```python
from build123d import *

# Parameters (mm, degrees)
SKETCH1_W                = 62
SKETCH1_H                = 26
BOSS_EXTRUDE1_DEPTH      = 6
SKETCH2_W                = 80
SKETCH2_H                = 10
BOSS_EXTRUDE2_DEPTH      = 50
M5_CLEARANCE_HOLE1_D     = 5.5
M5_CLEARANCE_HOLE1_DEPTH = 10
M5_CLEARANCE_HOLE1_TIP   = 1.652366702
BOSS_EXTRUDE3_DEPTH      = 9
BOSS_EXTRUDE4_START      = -80
BOSS_EXTRUDE4_DEPTH      = 9
M5_CLEARANCE_HOLE2_D     = 5.5
M5_CLEARANCE_HOLE2_DEPTH = 10
M5_CLEARANCE_HOLE2_TIP   = 1.652366702
FILLET1_R                = 3.5
FILLET2_R                = 1


with BuildPart() as part:
    # Sketch1 → Boss-Extrude1 (new body)
    with BuildSketch(Plane.XY):
        with Locations((31, 13)):
            Rectangle(SKETCH1_W, SKETCH1_H)
    extrude(amount=BOSS_EXTRUDE1_DEPTH)

    # Sketch2 → Boss-Extrude2 (add)
    with BuildSketch(Plane.XY.offset(6)):
        with Locations((31, 21)):
            Rectangle(SKETCH2_W, SKETCH2_H)
    extrude(amount=-BOSS_EXTRUDE2_DEPTH)

    # M5 Clearance Hole1
    with Locations(Plane(origin=(0, 0, 0), x_dir=(-1, 0, 0), z_dir=(0, 0, -1))):
        with Locations((-50.5, 8), (-11.5, 8)):
            Hole(M5_CLEARANCE_HOLE1_D / 2, depth=M5_CLEARANCE_HOLE1_DEPTH)
            with Locations((0, 0, -(M5_CLEARANCE_HOLE1_DEPTH + M5_CLEARANCE_HOLE1_TIP / 2))):  # 118° drill point
                Cone(0, M5_CLEARANCE_HOLE1_D / 2, M5_CLEARANCE_HOLE1_TIP, mode=Mode.SUBTRACT)

    # Sketch5 → Boss-Extrude3 (add)
    with BuildSketch(Plane(origin=(71, 0, 0), x_dir=(0, 0, -1), z_dir=(1, 0, 0))):
        Polygon((-6, 0), (10, 0), (44, 13), (44, 16), (-6, 16), align=None)
    extrude(amount=-BOSS_EXTRUDE3_DEPTH)

    # Sketch5<2> → Boss-Extrude4 (add)
    with BuildSketch(Plane(origin=(71, 0, 0), x_dir=(0, 0, -1), z_dir=(1, 0, 0)).offset(BOSS_EXTRUDE4_START)):
        Polygon((-6, 0), (10, 0), (44, 13), (44, 16), (-6, 16), align=None)
    extrude(amount=BOSS_EXTRUDE4_DEPTH)

    # M5 Clearance Hole2
    with Locations(Plane(origin=(0, 16, 0), x_dir=(-1, 0, 0), z_dir=(0, -1, 0))):
        with Locations((-38, 6), (-24, 6), (-56, 38), (-6, 38)):
            Hole(M5_CLEARANCE_HOLE2_D / 2, depth=M5_CLEARANCE_HOLE2_DEPTH)
            with Locations((0, 0, -(M5_CLEARANCE_HOLE2_DEPTH + M5_CLEARANCE_HOLE2_TIP / 2))):  # 118° drill point
                Cone(0, M5_CLEARANCE_HOLE2_D / 2, M5_CLEARANCE_HOLE2_TIP, mode=Mode.SUBTRACT)

    # Fillet1
    fillet1_edges = [part.edges().sort_by_distance(p)[0] for p in [
        (0, 8, 0),
        (62, 8, 0),
    ]]
    fillet(fillet1_edges, radius=FILLET1_R)

    # Fillet2
    fillet2_edges = [part.edges().sort_by_distance(p)[0] for p in [
        (0, 16, -23.75),
        (31, 16, 0),
        (1.025126266, 16, -1.025126266),
        (60.974873734, 16, -1.025126266),
        (62, 16, -23.75),
    ]]
    fillet(fillet2_edges, radius=FILLET2_R)


solid = part.part
```
Verification items for the finished model (mm, model axes). A direction names the side the tool comes from. Coordinates: 2 decimals unless noted, no trailing zeros. Write each loop counter-clockwise with the first axis right and the second up, starting at its lowest first coordinate (ties: lowest second). Pieces come first, ordered by that corner, then holes. Notation, with made-up numbers: M 45.25,-39.5 L 89.25,-39.5 A22 ccw 89.25,-6.5 Z; hole C -13.5,86 d8. An arc over 180 degrees is marked long. Answer as a JSON object with one key per item and string values. Group by question number.
(1) Cross-section at B-B, the plane z = -6. Record the cut outline in (x, y).
(2) Cross-section at D-D, the plane x = 16. Record the cut outline in (y, z).
(3) Cross-section at C-C, the plane y = 6.75. Record the cut outline in (x, z).
(4) Cross-section at A-A, the plane x = 6. Record the cut outline in (y, z), and give its area (3 significant figures).
(5) Gauge pin test, flat ends, axial feed: pin 1 (1.5 mm diameter, centred on x = 38, z = -31.5, fed in from -Y); pin 2 (4.5 mm diameter, centred on x = 26, y = 11, fed in from -Z). Record the tip position at first contact, or that the pin passes through.
(6) Material ranges on line 1 (X direction, y = 18.75, z = -38); line 2 (X direction, y = 9.5, z = -34); line 3 (Z direction, x = 38, y = 19.5), recorded low to high.
(7) Tool access check on faces 1 (the face through (31, 16, -22)), 2 (the face through (5.642, 21.07, -40.727)). Record the directions out of +Z, -Z, +X, -X, +Y, -Y that give a thin tool (end or side, any length) a straight path to the whole face; none if there is none.
(8) Release check for a two-part mould opening along Y. For faces 3 (the face through (30, 0, 2)), 4 (the face through (35.253, 21.07, -6.121)), 5 (the face through (14.04, 6.95, 3.04)) record: +Y half, -Y half, draft (parallel to the pull), parting line (faces both ways), or undercut.
Reply:
{
 "1": {"outline": "M -9,0 L 0,0 L 0,15 A1 cw 1,16 L 21.25,16 L 21.25,26 L -9,26 Z; M 26.75,16 L 35.25,16 L 35.25,26 L 26.75,26 Z; M 40.75,16 L 61,16 A1 cw 62,15 L 62,0 L 71,0 L 71,26 L 40.75,26 Z"},
 "2": {"outline": "M 0,0 L 15,0 A1 cw 16,-1 L 16,-44 L 26,-44 L 26,6 L 0,6 Z"},
 "3": {"outline": "M -9,-27.65 L 0,-27.65 L 0,-3.5 A3.5 cw 3.5,0 L 9.05,0 L 9.05,6 L -9,6 Z; M 13.95,0 L 48.05,0 L 48.05,6 L 13.95,6 Z; M 52.95,0 L 58.5,0 A3.5 cw 62,-3.5 L 62,-27.65 L 71,-27.65 L 71,6 L 52.95,6 Z"},
 "4": {"outline": "M 0,0 L 15,0 A1 cw 16,-1 L 16,-35.25 L 26,-35.25 L 26,6 L 0,6 Z; M 16,-44 L 26,-44 L 26,-40.75 L 16,-40.75 Z", "area": "541 mm²"},
 "5": {"pin 1": "y = 16", "pin 2": "z = 0"},
 "6": {"line 1": "-9 to 3.25, 8.75 to 53.25, 58.75 to 71", "line 2": "-9 to 0, 62 to 71", "line 3": "-44 to -8.75, -3.25 to 6"},
 "7": {"face 1": "-Z, -Y", "face 2": "+Y, -Y"},
 "8": {"face 3": "-Y half", "face 4": "draft", "face 5": "undercut"}
}
